Input: part model. Units: mm. Frame: model coordinates. Face numbers are marked on the shaded views. Coordinates: 2 decimals unless noted, no trailing zeros. Write each loop counter-clockwise with the first axis right and the second up, starting at its lowest first coordinate (ties: lowest second). Pieces come first, ordered by that corner, then holes. Notation, with made-up numbers: M 64,68 L 73,68 A10 cw 73,75 Z; hole C -21.5,10 d11. An arc over 180 degrees is marked long. Use CSV: the item, a comma, the result in double quotes.
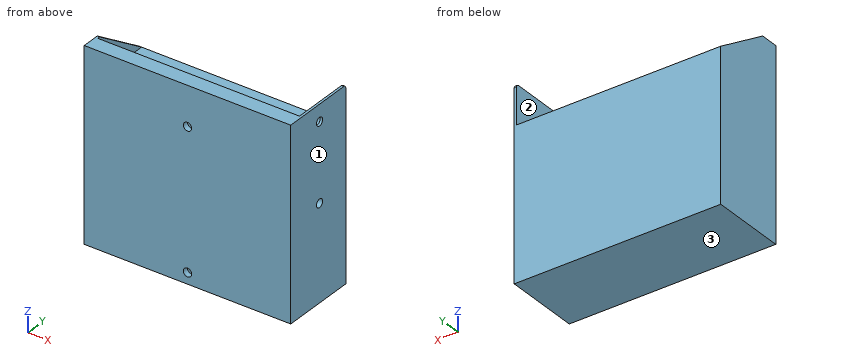
```python
from build123d import *

# Parameters (mm, degrees)
SKETCH1_W           = 74.25
SKETCH1_H           = 68.2
BOSS_EXTRUDE1_DEPTH = 27.2
SKETCH2_R           = 1.5
CUT_EXTRUDE1_DEPTH  = 10
SKETCH3_W           = 72.55
SKETCH3_H           = 14
CUT_EXTRUDE2_DEPTH  = 21.7
CHAMFER1_SIZE       = 14
CHAMFER1_SIZE2      = 20.755853559
FILLET1_R           = 1
SKETCH4_R           = 1.5
CUT_EXTRUDE3_DEPTH  = 2


with BuildPart() as part:
    # Sketch1 → Boss-Extrude1 (new body)
    with BuildSketch(Plane(origin=(0, 0, 0), x_dir=(1, 0, 0), z_dir=(0, 1, 0))):
        Rectangle(SKETCH1_W, SKETCH1_H)
    extrude(amount=BOSS_EXTRUDE1_DEPTH)

    # Sketch2 → Cut-Extrude1 (cut)
    with BuildSketch(Plane(origin=(37.125, 0, 0), x_dir=(0, 0, -1), z_dir=(1, 0, 0))):
        with Locations((-28.1, 14.25)):
            Circle(SKETCH2_R)
        with Locations((-0.1, 14.25)):
            Circle(SKETCH2_R)
    extrude(amount=-CUT_EXTRUDE1_DEPTH, mode=Mode.SUBTRACT)

    # Sketch3 → Cut-Extrude2 (cut)
    with BuildSketch(Plane(origin=(0, 27.2, 0), x_dir=(1, 0, 0), z_dir=(0, 1, 0))):
        with Locations((0, -27.1)):
            Rectangle(SKETCH3_W, SKETCH3_H)
    extrude(amount=-CUT_EXTRUDE2_DEPTH, mode=Mode.SUBTRACT)

    # Chamfer1
    chamfer1_edges = [part.edges().sort_by_distance(p)[0] for p in [
        (-36.7, 27.2, 34.1),
    ]]
    chamfer1_side = [part.faces().sort_by_distance(p)[0] for p in [
        (0, 27.2, -6.799518298),
    ]]
    chamfer(chamfer1_edges, length=CHAMFER1_SIZE, length2=CHAMFER1_SIZE2, reference=chamfer1_side[0])

    # Fillet1
    fillet1_edges = [part.edges().sort_by_distance(p)[0] for p in [
        (36.7, 27.2, 34.1),
    ]]
    fillet(fillet1_edges, radius=FILLET1_R)

    # Sketch4 → Cut-Extrude3 (cut)
    with BuildSketch(Plane.XZ):
        with Locations(Location((0, -30.1, 0), (0, 0, 270))):
            Circle(SKETCH4_R)
        with Locations(Location((0, 19.9, 0), (0, 0, 270))):
            Circle(SKETCH4_R)
    extrude(amount=-CUT_EXTRUDE3_DEPTH, mode=Mode.SUBTRACT)


solid = part.part
```
1. Section C-C (y = 25). Return loops of the section in (x, z) (3 decimals), then the cut area to 3 significant figures.
Resolved:
outline,"M -37.125,-34.1 L 37.125,-34.1 L 37.125,34.1 L 36.275,34.1 L 36.275,20.1 L -36.275,20.1 L -36.275,21.584 L -37.125,21.584 Z"
area,"4,040 mm^2"
2. Section A-A (x = 0). Return loops of the section in (y, z), then the cut area to 3 significant figures.
Resolved:
outline,"M 0,-34.1 L 27.2,-34.1 L 27.2,20.1 L 5.5,20.1 L 5.5,34.1 L 0,34.1 L 0,21.4 L 2,21.4 L 2,18.4 L 0,18.4 L 0,-28.6 L 2,-28.6 L 2,-31.6 L 0,-31.6 Z"
area,"1,540 mm^2"
3. Section D-D (y = 11.75). Return loops of the section in (x, z) (3 decimals).
Resolved:
outline,"M -37.125,-34.1 L 37.125,-34.1 L 37.125,34.1 L 36.275,34.1 L 36.275,20.1 L -36.275,20.1 L -36.275,30.521 L -37.125,30.521 Z"
4. Contact query for flat-ended pins moving along their axis: pin 1 Ø2 at (x, y) = (24, 18.5) entering from +Z; pin 2 Ø5 at (x, z) = (19, -1) entering from -Y; pin 3 Ø11 at (x, z) = (10.5, 27.5) entering from +Y; pin 4 Ø1.8 at (y, z) = (14.25, 0.1) entering from +X (3 decimals). Output: stop coordinate, or through.
Resolved:
pin 1,"stops at z = 20.1"
pin 2,"stops at y = 0"
pin 3,"stops at y = 5.5"
pin 4,"stops at x = 27.125"
5. Material intervals for line 1 (X direction, y = 0.9, z = 19.9) (3 decimals); line 2 (Y direction, x = 36.85, z = 28.1); line 3 (Z direction, x = 1, y = 13.75), sorted ascending. Write a range as [from, to].
Resolved:
line 1,"x = [-37.125, -1.5], [1.5, 37.125]"
line 2,"y = [0, 12.75], [15.75, 27.2]"
line 3,"z = [-34.1, 20.1]"
6. Mould query, pull axis X, two halves, no side actions, for the marked faces 1, 2 and 3. Classes: pulls with the +X half, pulls with the -X half, needs draft (parallel to the pull), parting line crosses it, or undercut.
Resolved:
face 1,"pulls with the +X half"
face 2,"undercut"
face 3,"needs draft"
7. Section B-B (z = 28.1). Return loops of the section in (x, y) (3 decimals), then the cut area to 3 significant figures.
Resolved:
outline,"M -37.125,0 L 37.125,0 L 37.125,12.75 L 36.275,12.75 L 36.275,5.5 L -36.275,5.5 L -36.275,15.34 L -37.125,15.34 Z; M 36.275,15.75 L 37.125,15.75 L 37.125,27.2 L 36.275,27.2 Z"
area,"433 mm^2"
